```python
from build123d import *

# Parameters (mm, degrees)
CROQUIS1_W              = 8
CROQUIS1_H              = 10
CROQUIS1_R              = 1.5
SALIENTE_EXTRUIR1_DEPTH = 2
ESCALA1_SCALE           = 7


with BuildPart() as part:
    # Croquis1 → Saliente-Extruir1 (new body)
    with BuildSketch(Plane(origin=(0, 0, 0), x_dir=(1, 0, 0), z_dir=(0, 1, 0))):
        with Locations((4, -5)):
            Rectangle(CROQUIS1_W, CROQUIS1_H)
        with Locations((4.048599745, -8.17997322)):
            Circle(CROQUIS1_R, mode=Mode.SUBTRACT)
    extrude(amount=SALIENTE_EXTRUIR1_DEPTH)


with BuildPart() as part_1:
    # Escala1: scaled about (3.995289666, 1, 4.691793918)
    add(part.part.scale(ESCALA1_SCALE).moved(Location((-23.971737996, -6, -28.150763508))))


solid = part_1.part
```
Check sheet for the modelled part. Datum: model origin and axes. Units: mm. Round coordinates to 2 decimals unless told otherwise and drop trailing zeros. Order: outer loops, then holes, each group sorted by start corner. A loop starts at its lowest first (then second) coordinate and runs counter-clockwise, first axis right, second up. Notation, with made-up numbers: M 74,14 L 112,14 A29 ccw 112,35 Z; hole C 6,65.5 d1. An arc over 180 degrees is marked long. Answer in a Markdown table with one row per item.
(1) Material ranges on line 1 along X through (y, z) = (0.5, 29); line 2 along Z through (x, y) = (11.5, 3.25); line 3 along Z through (x, y) = (8.5, 3.5), recorded low to high. Write a range as from..to.
Findings:
| item | result |
|---|---|
| line 1 | x = -23.97..-6.13, 14.87..32.03 |
| line 2 | z = -28.15..21.4, 36.82..41.85 |
| line 3 | z = -28.15..19.46, 38.76..41.85 |
(2) Section check C-C on y = 7. Record the boundary of the cut face in (x, z), plus the area to 3 significant figures.
Findings:
| item | result |
|---|---|
| outline | M -23.97,-28.15 L 32.03,-28.15 L 32.03,41.85 L -23.97,41.85 Z; hole C 4.37,29.11 d21 |
| area | 3,570 mm^2 |
(3) Section check B-B on x = 12. Record the boundary of the cut face in (y, z), plus the area to 3 significant figures.
Findings:
| item | result |
|---|---|
| outline | M -6,-28.15 L 8,-28.15 L 8,21.9 L -6,21.9 Z; M -6,36.32 L 8,36.32 L 8,41.85 L -6,41.85 Z |
| area | 778 mm^2 |
(4) Draft check along X on faces 1 (the flat face through (32.028, 1, 7)), 2 (the flat face through (-23.972, 1, 7)), 3 (the flat face through (4, 1, 41.849)), 4 (the cylindrical face through (3, 0.9, 18.7)). Enter one of: +X half, -X half, draft (parallel to the pull), parting line (faces both ways), or undercut.
Findings:
| item | result |
|---|---|
| face 1 | +X half |
| face 2 | -X half |
| face 3 | draft |
| face 4 | undercut |
(5) Section check A-A on z = 27. Record the boundary of the cut face in (x, y).
Findings:
| item | result |
|---|---|
| outline | M -23.97,-6 L -5.92,-6 L -5.92,8 L -23.97,8 Z; M 14.65,-6 L 32.03,-6 L 32.03,8 L 14.65,8 Z |
